```python
from build123d import *

# Parameters (mm, degrees)
SKETCH1_W           = 57
SKETCH1_H           = 57
BOSS_EXTRUDE1_DEPTH = 57
SKETCH2_R           = 2.55
CUT_EXTRUDE1_DEPTH  = 58
CUT_EXTRUDE2_DEPTH  = 53.34
SKETCH4_R           = 19.05
BOSS_EXTRUDE2_DEPTH = 1.6
SKETCH5_R           = 3.175
BOSS_EXTRUDE3_DEPTH = 19.4
CUT_EXTRUDE3_DEPTH  = 15
CHAMFER1_SIZE2      = 0.439940905
CHAMFER1_SIZE       = 0.254
FILLET1_R           = 2.54
FILLET2_R           = 0.508


with BuildPart() as part:
    # Sketch1 → Boss-Extrude1 (new body)
    with BuildSketch(Plane.XY):
        Rectangle(SKETCH1_W, SKETCH1_H)
    extrude(amount=BOSS_EXTRUDE1_DEPTH)

    # Sketch2 → Cut-Extrude1 (cut, through all)
    with BuildSketch(Plane.XY.offset(57)):
        with Locations((-23.5, 23.5)):
            Circle(SKETCH2_R)
        with Locations((23.5, 23.5)):
            Circle(SKETCH2_R)
        with Locations((23.5, -23.5)):
            Circle(SKETCH2_R)
        with Locations((-23.5, -23.5)):
            Circle(SKETCH2_R)
    extrude(amount=-CUT_EXTRUDE1_DEPTH, mode=Mode.SUBTRACT)

    # Sketch3 → Cut-Extrude2 (cut)
    with BuildSketch(Plane.XY.offset(57)):
        with BuildLine():
            Line((-18.5, 23.5), (-18.5, 28.5))
            Line((-18.5, 28.5), (-28.5, 28.5))
            Line((-28.5, 28.5), (-28.5, 18.5))
            Line((-28.5, 18.5), (-23.5, 18.5))
            ThreePointArc((-23.5, 18.5), (-19.964466094, 19.964466094), (-18.5, 23.5))
        make_face()
        with BuildLine():
            Line((28.5, 28.5), (28.5, 18.5))
            Line((28.5, 18.5), (23.5, 18.5))
            ThreePointArc((23.5, 18.5), (19.964466094, 19.964466094), (18.5, 23.5))
            Line((18.5, 23.5), (18.5, 28.5))
            Line((18.5, 28.5), (28.5, 28.5))
        make_face()
        with BuildLine():
            Line((-28.5, -28.5), (-28.5, -18.5))
            Line((-28.5, -18.5), (-23.5, -18.5))
            ThreePointArc((-23.5, -18.5), (-19.964466094, -19.964466094), (-18.5, -23.5))
            Line((-18.5, -23.5), (-18.5, -28.5))
            Line((-18.5, -28.5), (-28.5, -28.5))
        make_face()
        with BuildLine():
            Line((18.5, -23.5), (18.5, -28.5))
            Line((18.5, -28.5), (28.5, -28.5))
            Line((28.5, -28.5), (28.5, -18.5))
            Line((28.5, -18.5), (23.5, -18.5))
            ThreePointArc((23.5, -18.5), (19.964466094, -19.964466094), (18.5, -23.5))
        make_face()
    extrude(amount=-CUT_EXTRUDE2_DEPTH, mode=Mode.SUBTRACT)

    # Sketch4 → Boss-Extrude2 (add)
    with BuildSketch(Plane(origin=(0, 0, 0), x_dir=(-1, 0, 0), z_dir=(0, 0, -1))):
        Circle(SKETCH4_R)
    extrude(amount=BOSS_EXTRUDE2_DEPTH)

    # Sketch5 → Boss-Extrude3 (add)
    with BuildSketch(Plane(origin=(0, 0, -1.6), x_dir=(-1, 0, 0), z_dir=(0, 0, -1))):
        Circle(SKETCH5_R)
    extrude(amount=BOSS_EXTRUDE3_DEPTH)

    # Sketch7 → Cut-Extrude3 (cut)
    with BuildSketch(Plane(origin=(0, 0, -21), x_dir=(-1, 0, 0), z_dir=(0, 0, -1))):
        with BuildLine():
            Line((-1.234908904, 2.925), (-1.234908904, -2.925))
            ThreePointArc((-1.234908904, -2.925), (-3.175, 0), (-1.234908904, 2.925))
        make_face()
    extrude(amount=-CUT_EXTRUDE3_DEPTH, mode=Mode.SUBTRACT)

    # Chamfer1
    chamfer1_edges = [part.edges().sort_by_distance(p)[0] for p in [
        (-1.754962853, -2.645889337, -21),
    ]]
    chamfer(chamfer1_edges, length=CHAMFER1_SIZE, length2=CHAMFER1_SIZE2)

    # Fillet1
    fillet1_edges = [part.edges().sort_by_distance(p)[0] for p in [
        (-28.5, 28.5, 1.83),
        (28.5, -28.5, 1.83),
        (-28.5, -28.5, 1.83),
        (28.5, 28.5, 1.83),
    ]]
    fillet(fillet1_edges, radius=FILLET1_R)

    # Fillet2
    fillet2_edges = [part.edges().sort_by_distance(p)[0] for p in [
        (-28.5, 0, 57),
        (-19.964466094, 19.964466094, 57),
        (-18.5, 26, 57),
        (-26, 18.5, 57),
        (-28.5, 18.5, 30.33),
        (-18.5, 28.5, 30.33),
        (0, -28.5, 57),
        (28.5, 0, 57),
        (0, 28.5, 57),
        (19.964466094, 19.964466094, 57),
        (26, 18.5, 57),
        (18.5, 26, 57),
        (18.5, 28.5, 30.33),
        (28.5, 18.5, 30.33),
        (-19.964466094, -19.964466094, 57),
        (-26, -18.5, 57),
        (-18.5, -26, 57),
        (-18.5, -28.5, 30.33),
        (-28.5, -18.5, 30.33),
        (19.964466094, -19.964466094, 57),
        (18.5, -26, 57),
        (26, -18.5, 57),
        (28.5, -18.5, 30.33),
        (18.5, -28.5, 30.33),
    ]]
    fillet(fillet2_edges, radius=FILLET2_R)


solid = part.part
```
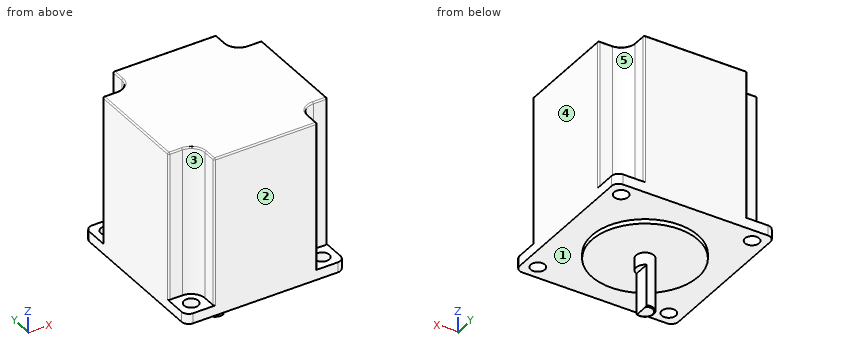
Geometry check sheet. Reference: the model listing, model coordinates, mm. Face numbers are marked on the shaded views. A direction names the side the tool comes from. Give positions to 0.01 mm unless a question says otherwise; leave off trailing zeros. Write each loop counter-clockwise with the first axis right and the second up, starting at its lowest first coordinate (ties: lowest second). Pieces come first, ordered by that corner, then holes. Notation, with made-up numbers: (-3, 25.25) - (34, 25.25) arc R17 ccw to (34, 46.25) - close; hole circle Ø5 at (-6, 83.5). An arc over 180 degrees is marked (long way). Use a Markdown table: item, result.
Q1. Section check B-B, the plane z = 25. Enter the section's corners in (x, y), then the cut area to 3 significant figures.
Computed:
| item | result |
|---|---|
| outline | (-28.5, -17.99) arc R0.51 ccw to (-27.99, -18.5) - (-23.5, -18.5) arc R5 cw to (-18.5, -23.5) - (-18.5, -27.99) arc R0.51 ccw to (-17.99, -28.5) - (17.99, -28.5) arc R0.51 ccw to (18.5, -27.99) - (18.5, -23.5) arc R5 cw to (23.5, -18.5) - (27.99, -18.5) arc R0.51 ccw to (28.5, -17.99) - (28.5, 17.99) arc R0.51 ccw to (27.99, 18.5) - (23.5, 18.5) arc R5 cw to (18.5, 23.5) - (18.5, 27.99) arc R0.51 ccw to (17.99, 28.5) - (-17.99, 28.5) arc R0.51 ccw to (-18.5, 27.99) - (-18.5, 23.5) arc R5 cw to (-23.5, 18.5) - (-27.99, 18.5) arc R0.51 ccw to (-28.5, 17.99) - close |
| area | 2,870 mm² |
Q2. Section check A-A, the plane y = 0. Enter the section's corners in (x, z) (3 decimals), then the cut area to 3 significant figures.
Computed:
| item | result |
|---|---|
| outline | (-28.5, 0) - (-19.05, 0) - (-19.05, -1.6) - (-3.175, -1.6) - (-3.175, -20.746) - (-2.735, -21) - (1.235, -21) - (1.235, -6) - (3.175, -6) - (3.175, -1.6) - (19.05, -1.6) - (19.05, 0) - (28.5, 0) - (28.5, 56.492) arc R0.508 ccw to (27.992, 57) - (-27.992, 57) arc R0.508 ccw to (-28.5, 56.492) - close |
| area | 3,400 mm² |
Q3. Set-up check for the marked faces 1, 2, 3, 4 and 5: record each of +Z, -Z, +X, -X, +Y, -Y from which the full face is reachable in a straight line by a thin tool's end or side.
Computed:
| item | result |
|---|---|
| face 1 | -Z |
| face 2 | +Z, -Z, +X, -X, -Y |
| face 3 | +Z, -X, -Y |
| face 4 | +Z, -Z, +X, +Y, -Y |
| face 5 | +Z, +X, +Y |
Q4. Go/stop test with flat-tipped pins: P1, Ø0.6, axis at x = 2, y = 0, coming from the -Z side; P2, Ø3.5, axis at y = 25, z = 35.5, coming from the +X side; P3, Ø1, axis at y = 0, z = -6.5, coming from the -X side (3 decimals). Record where each tip stops, or that it passes through.
Computed:
| item | result |
|---|---|
| P1 | stops at z = -6 |
| P2 | stops at x = 18.51 |
| P3 | stops at x = -3.175 |
Q5. Thickness scan on L1, parallel to Y at x = 23.5, z = 2.3; L2, parallel to Z at x = 26.5, y = 2.5; L3, parallel to Z at x = 6, y = 4. Record the ranges inside material, lowest first. Write a range as [from, to].
Computed:
| item | result |
|---|---|
| L1 | y = [-28.5, -26.05], [-20.95, 20.95], [26.05, 28.5] |
| L2 | z = [0, 57] |
| L3 | z = [-1.6, 57] |
Q6. Section check C-C, the plane x = 0. Enter the section's corners in (y, z) (3 decimals), then the cut area to 3 significant figures.
Computed:
| item | result |
|---|---|
| outline | (-28.5, 0) - (-19.05, 0) - (-19.05, -1.6) - (-3.175, -1.6) - (-3.175, -20.746) - (-2.735, -21) - (2.735, -21) - (3.175, -20.746) - (3.175, -1.6) - (19.05, -1.6) - (19.05, 0) - (28.5, 0) - (28.5, 56.492) arc R0.508 ccw to (27.992, 57) - (-27.992, 57) arc R0.508 ccw to (-28.5, 56.492) - close |
| area | 3,430 mm² |
Q7. Section check D-D, the plane x = 6. Enter the section's corners in (y, z), then the cut area to 3 significant figures.
Computed:
| item | result |
|---|---|
| outline | (-28.5, 0) - (-18.08, 0) - (-18.08, -1.6) - (18.08, -1.6) - (18.08, 0) - (28.5, 0) - (28.5, 56.49) arc R0.51 ccw to (27.99, 57) - (-27.99, 57) arc R0.51 ccw to (-28.5, 56.49) - close |
| area | 3,310 mm² |
